Source: CAD feature listing. Evaluate the final solid. Frame: model axes, mm. A direction names the side the tool comes from. Round coordinates to 2 decimals unless told otherwise and drop trailing zeros. Order: outer loops, then holes, each group sorted by start corner. A loop starts at its lowest first (then second) coordinate and runs counter-clockwise, first axis right, second up. Notation, with made-up numbers: M -36.5,82 L -0.5,82 A17 cw -0.5,110 Z; hole C 21,-39 d3. An arc over 180 degrees is marked long. Answer as CSV lines item,"result". Start each with the question number.
Item 1: Pull-direction query (Y, two-part tool) for faces 4 (the face through (52.423, -21.578, 33.031)), 5 (the face through (0.907, -96.148, 33.031)), 6 (the face through (50.665, 23.561, 33.031)), 7 (the face through (-1, 0, 0)); classes: +Y half, -Y half, draft (parallel to the pull), parting line (faces both ways), or undercut.
Item 2: Section query D-D on y = -4. Return the cut outline in (x, z) (3 decimals), plus the area to 3 significant figures.
Item 3: Section query C-C on z = 62.5. Return the cut outline in (x, y), plus the area to 3 significant figures.
Item 4: First-contact query: P1, Ø3, axis at x = -44, z = 60.5, coming from the -Y side; P2, Ø2, axis at y = -5, z = 20.5, coming from the +X side; P3, Ø8, axis at y = -65, z = 59, coming from the +X side (3 decimals). Flat tips, straight axial feed; report the tip coordinate or a pass-through.
Item 5: Line query: line 1 (X direction, y = -69, z = 7.5); line 2 (Y direction, x = -52, z = 6.5); line 3 (Y direction, x = 32.5, z = 28). Output: solid intervals per line, ascending. Write a range as [from, to].
Item 6: Section query B-B on y = 36. Return the cut outline in (x, z) (3 decimals), plus the area to 3 significant figures.
Item 7: Section query A-A on z = 29.5. Return the cut outline in (x, y), plus the area to 3 significant figures.
Item 8: Set-up query: faces 1 (the face through (-0.84, 93.51, 33.03)), 2 (the face through (-50.59, 23.484, 33.031)), 3 (the face through (-1, 0, 67)). Return all of +Z, -Z, +X, -X, +Y, -Y with unobstructed straight access to the full face (end or side cutting, diameter ignored); none if empty.
Autodesk Inventor part; units mm, degrees
ref_plane "EPDOPPELNUT2_XY" through (0, 47.88, 0) normal (0, 0, 1) x (1, 0, 0)
ref_plane "EPDOPPELNUT2_YZ" through (0, 47.88, 0) normal (1, 0, 0) x (0, 1, 0)
ref_plane "EPDOPPELNUT2_ZX" through (0, 47.88, 0) normal (0, 1, 0) x (0, 0, 1)
sketch "Skizze_1" plane through (0, 0, 0) normal (0, 0, 1) x (1, 0, 0)
  line L0 (-57.155, -41.88) -> (-57.055, -41.88)
  line L1 (-57.055, -41.88) -> (-57.055, -53.88)
  line L2 (-57.055, -53.88) -> (-57.155, -53.88)
  line L3 (-57.155, -53.88) -> (-57.155, -69.7905)
  arc A0 (-57.155, -69.7905) -> (57.155, -69.7905) centre (0, -22.63) ccw
  line L4 (57.155, -69.7905) -> (57.155, -53.88)
  line L5 (57.155, -53.88) -> (57.055, -53.88)
  line L6 (57.055, -53.88) -> (57.055, -41.88)
  line L7 (57.055, -41.88) -> (57.155, -41.88)
  line L8 (57.155, -41.88) -> (57.155, -25.9695)
  arc A1 (57.155, -25.9695) -> (48.655, -17.2417) centre (0, -73.13) ccw
  line L9 (48.655, -17.2417) -> (48.655, 20.7961)
  arc A2 (48.655, 20.7961) -> (53.655, 25.9369) centre (0, 73.12) ccw
  line L10 (53.655, 25.9369) -> (53.655, 41.88)
  line L11 (53.655, 41.88) -> (53.555, 41.88)
  line L12 (53.555, 41.88) -> (53.555, 53.88)
  line L13 (53.555, 53.88) -> (53.655, 53.88)
  line L14 (53.655, 53.88) -> (53.655, 69.8231)
  arc A3 (53.655, 69.8231) -> (-53.655, 69.8231) centre (0, 22.64) ccw
  line L15 (-53.655, 69.8231) -> (-53.655, 53.88)
  line L16 (-53.655, 53.88) -> (-53.555, 53.88)
  line L17 (-53.555, 53.88) -> (-53.555, 41.88)
  line L18 (-53.555, 41.88) -> (-53.655, 41.88)
  line L19 (-53.655, 41.88) -> (-53.655, 25.9369)
  arc A4 (-53.655, 25.9369) -> (-48.655, 20.7961) centre (0, 73.12) ccw
  line L20 (-48.655, 20.7961) -> (-48.655, -17.2417)
  arc A5 (-48.655, -17.2417) -> (-57.155, -25.9695) centre (0, -73.13) ccw
  line L21 (-57.155, -25.9695) -> (-57.155, -41.88)
extrude "Extrusion1" add sketch "Skizze_1" along normal blind 67 draft -1
ref_plane "EPDOPPELNUT2_XY" through (0, 47.88, 0) normal (0, 0, 1) x (1, 0, 0)
ref_plane "EPDOPPELNUT2_YZ" through (0, 47.88, 0) normal (1, 0, 0) x (0, 1, 0)
ref_plane "EPDOPPELNUT2_ZX" through (0, 47.88, 0) normal (0, 1, 0) x (0, 0, 1)
ref_plane "EPDOPPROFIL_XY" through (0, 47.88, 67) normal (0, 0, 1) x (1, 0, 0)
ref_plane "EPDOPPROFIL_YZ" through (0, 47.88, 67) normal (1, 0, 0) x (0, 1, 0)
ref_plane "EPDOPPROFIL_ZX" through (0, 47.88, 67) normal (0, 1, 0) x (0, 0, 1)
ref_plane "EPFUNKTIONSPR2_XY" through (0, -47.88, 0) normal (0, 0, 1) x (1, 0, 0)
ref_plane "EPFUNKTIONSPR2_YZ" through (0, -47.88, 0) normal (1, 0, 0) x (0, 1, 0)
ref_plane "EPFUNKTIONSPR2_ZX" through (0, -47.88, 0) normal (0, 1, 0) x (0, 0, 1)
ref_plane "EPKONPROFIL_XY" through (0, -47.88, 67) normal (0, 0, 1) x (1, 0, 0)
ref_plane "EPKONPROFIL_YZ" through (0, -47.88, 67) normal (1, 0, 0) x (0, 1, 0)
ref_plane "EPKONPROFIL_ZX" through (0, -47.88, 67) normal (0, 1, 0) x (0, 0, 1)
properties part number "LZ80_Gehaeuse_Parallelform"
Results:
1,face 4,"undercut"
1,face 5,"-Y half"
1,face 6,"undercut"
1,face 7,"draft"
2,outline,"M -48.655,0 L 48.655,0 L 47.486,67 L -47.486,67 Z"
2,area,"6,440 mm^2"
3,outline,"M -56.06,-69.4 A73.01 ccw 56.06,-69.4 L 56.06,-54.97 L 55.96,-54.97 L 55.96,-40.79 L 56.06,-40.79 L 56.06,-26.36 A73.01 ccw 47.56,-17.74 L 47.56,21.27 A70.37 ccw 52.56,26.35 L 52.56,40.79 L 52.46,40.79 L 52.46,54.97 L 52.56,54.97 L 52.56,69.41 A70.36 ccw -52.56,69.41 L -52.56,54.97 L -52.46,54.97 L -52.46,40.79 L -52.56,40.79 L -52.56,26.35 A70.35 ccw -47.56,21.27 L -47.56,-17.74 A73 ccw -56.06,-26.36 L -56.06,-40.79 L -55.96,-40.79 L -55.96,-54.97 L -56.06,-54.97 Z"
3,area,"18,200 mm^2"
4,P1,"y = -82.04"
4,P2,"x = 48.31"
4,P3,"x = 56.195"
5,line 1,"[-57.02, 57.02]"
5,line 2,"[-75.26, -20.5], [24.28, 71.48]"
5,line 3,"[-88.68, 85.72]"
6,outline,"M -53.655,0 L 53.655,0 L 52.486,67 L -52.486,67 Z"
6,area,"7,110 mm^2"
7,outline,"M -56.64,-69.61 A73.59 ccw 56.64,-69.61 L 56.64,-54.39 L 56.54,-54.39 L 56.54,-41.37 L 56.64,-41.37 L 56.64,-26.15 A73.59 ccw 48.14,-17.48 L 48.14,21.02 A70.95 ccw 53.14,26.13 L 53.14,41.37 L 53.04,41.37 L 53.04,54.39 L 53.14,54.39 L 53.14,69.63 A70.94 ccw -53.14,69.63 L -53.14,54.39 L -53.04,54.39 L -53.04,41.37 L -53.14,41.37 L -53.14,26.13 A70.92 ccw -48.14,21.02 L -48.14,-17.48 A73.58 ccw -56.64,-26.15 L -56.64,-41.37 L -56.54,-41.37 L -56.54,-54.39 L -56.64,-54.39 Z"
7,area,"18,500 mm^2"
8,face 1,"+Z, +Y"
8,face 2,"+Z, -X"
8,face 3,"+Z, +X, -X, +Y, -Y"
